Source: CAD feature listing. Evaluate the final solid. Frame: model axes, mm. A direction names the side the tool comes from. Coordinates: 2 decimals unless noted, no trailing zeros. Loops run counter-clockwise (first coordinate to the right, second up) from the corner with the lowest first, then second, coordinate; pieces in that order, holes last.
Solid Edge part; units mm, degrees
sketch "Sketch1" plane through (0, 0, 0) normal (1, 0, 0) x (0, 1, 0)
  line L0 (-12.5363, -10.0816) -> (15.4637, -10.0816)
  line L1 (15.4637, -10.0816) -> (15.4637, 4.9184)
  line L2 (15.4637, 4.9184) -> (-12.5363, 4.9184)
  line L3 (-12.5363, 4.9184) -> (-12.5363, -10.0816)
  dimension "D1" = 12.5363
  dimension "D2" = 12.5363
extrude "Protrusion1" add sketch "Sketch1" against normal blind 3
sketch "Sketch2" plane through (-3, 1.4637, -2.5816) normal (-1, 0, 0) x (0, 1, 0)
  line L0 (14, 7.5) -> (11, 7.5)
  line L1 (11, 7.5) -> (11, -7.5388)
  line L2 (11, -7.5388) -> (14, -7.5388)
  line L3 (14, -7.5388) -> (14, 7.5)
extrude "ProtrusiónExtruida_8" add sketch "Sketch2" along normal blind 35
sketch "Sketch3" plane through (-3, -0.0363, -2.5816) normal (-1, 0, 0) x (0, 1, 0)
  line L0 (-12.5, 7.5) -> (-9.5, 7.5)
  line L1 (-9.5, 7.5) -> (-9.5, -7.5)
  line L2 (-9.5, -7.5) -> (-12.5, -7.5)
  line L3 (-12.5, -7.5) -> (-12.5, 7.5)
extrude "ProtrusiónExtruida_9" add sketch "Sketch3" along normal blind 20
sketch "Sketch4" plane through (-19, 15.4637, -2.5622) normal (0, 1, 0) x (0, 0, -1)
  circle A0 centre (-0.0194, 0) radius 1.5
extrude "VaciadoExtruido_2" cut sketch "Sketch4" against normal blind 13.4467
fillet "Redondeo_1" radius 3 1 edges at (-17.5, 12.4637, -2.5429)
Q1. Section A-A, the plane x = -19. Count the separate pieces of the cut face and the enclosed holes in it, plus the area to 3 significant figures.
Q2. Section D-D, the plane y = -6.75. Return the cut outline in (x, z).
Q3. Line query: line 1 along Y through (x, z) = (-11, -7.5); line 2 along Y through (x, z) = (-28, -2.5); line 3 along X through (y, z) = (-2.75, -4). Output: solid intervals per line, ascending.
Q4. Section B-B, the plane z = -7.5. Return the cut outline in (x, y), plus the area to 3 significant figures.
Q5. Contact query for flat-ended pins moving along their axis: pin 1 Ø2.5 at (y, z) = (-11.5, -6) entering from -X; pin 2 Ø12 at (x, y) = (-27, -6) entering from +Z; pin 3 Ø2 at (y, z) = (0.5, -5.5) entering from -X. Output: stop coordinate, or through.
Q6. Access query for faces 1 (the flat face through (-23, -11, -3)), 2 (the flat face through (-12, 13, -10.082)), 3 (the flat face through (-13, -9.536, -3)). Directions: +Z, -Z, +X, -X, +Y, -Y. A direction counts if a zero-diameter tool reaches every point of the face in a straight line with its end or side. Return the directions, or none.
Derived:
1. separate pieces: 3
1. enclosed holes: 0
1. area: 77.3 mm2
2. outline: (-3, -10.08) - (0, -10.08) - (0, 4.92) - (-3, 4.92) - close
3. line 1: y = -12.54 to -9.54, 12.46 to 15.46
3. line 2: y = 12.46 to 15.46
3. line 3: x = -3 to 0
4. outline: (-38, 12.46) - (-3, 12.46) - (-3, -9.54) - (-23, -9.54) - (-23, -12.54) - (0, -12.54) - (0, 15.46) - (-38, 15.46) - close
4. area: 249 mm2
5. pin 1: stops at x = -23
5. pin 2: stops at z = 4.92
5. pin 3: stops at x = -3
6. face 1: +Z, -Z, -X, -Y
6. face 2: -Z, +X, -X, +Y, -Y
6. face 3: +Z, -Z, -X
